```python
from build123d import *

# Parameters (mm, degrees)
BOSS_EXTRUDE1_DEPTH   = 79.375
BOSS_EXTRUDE1_2_DEPTH = 79.375
BOSS_EXTRUDE2_DEPTH   = 3.175
BOSS_EXTRUDE3_START   = 3.175
BOSS_EXTRUDE3_DEPTH   = 3.175


with BuildPart() as part:
    # Sketch2 → Boss-Extrude1 (new body)
    with BuildSketch(Plane.XY):
        with BuildLine():
            Line((0, 304.8), (0, 307.975))
            ThreePointArc((0, 307.975), (-56.126600757, 284.726600757), (-79.375, 228.6))
            Line((-79.375, 228.6), (-79.375, 76.2))
            ThreePointArc((-79.375, 76.2), (-63.5, 28.575), (-22.225, 0))
            Line((-22.225, 0), (0, 0))
            ThreePointArc((0, 0), (-53.881536726, 22.318463274), (-76.2, 76.2))
            Line((-76.2, 76.2), (-76.2, 228.6))
            ThreePointArc((-76.2, 228.6), (-53.881536726, 282.481536726), (0, 304.8))
        make_face()
    extrude(amount=BOSS_EXTRUDE1_DEPTH)



with BuildPart() as body_2:
    # Sketch2 → Boss-Extrude1 2 (new body)
    with BuildSketch(Plane.XY):
        with BuildLine():
            ThreePointArc((-48.2, 88.2), (-34.082546853, 54.117453147), (0, 40))
            Line((0, 40), (0, 43.175))
            ThreePointArc((0, 43.175), (-31.837482823, 56.362517177), (-45.025, 88.2))
            Line((-45.025, 88.2), (-45.025, 216.6))
            ThreePointArc((-45.025, 216.6), (-31.837482823, 248.437482823), (0, 261.625))
            Line((0, 261.625), (0, 264.8))
            ThreePointArc((0, 264.8), (-34.082546853, 250.682546853), (-48.2, 216.6))
            Line((-48.2, 216.6), (-48.2, 88.2))
        make_face()
    extrude(amount=BOSS_EXTRUDE1_2_DEPTH)


with BuildPart() as part_1:
    add(part.part)

    add(body_2.part)  # Boss-Extrude2 merges body 2
    # Sketch3 → Boss-Extrude2 (add)
    with BuildSketch(Plane.XY.offset(79.375)):
        with BuildLine():
            Line((-45.025, 88.2), (-45.025, 216.6))
            ThreePointArc((-45.025, 216.6), (-31.837482823, 248.437482823), (0, 261.625))
            Line((0, 261.625), (0, 307.975))
            ThreePointArc((0, 307.975), (-56.126600757, 284.726600757), (-79.375, 228.6))
            Line((-79.375, 228.6), (-79.375, 76.2))
            ThreePointArc((-79.375, 76.2), (-63.5, 28.575), (-22.225, 0))
            Line((-22.225, 0), (0, 0))
            Line((0, 0), (0, 43.175))
            ThreePointArc((0, 43.175), (-31.837482823, 56.362517177), (-45.025, 88.2))
        make_face()
    extrude(amount=BOSS_EXTRUDE2_DEPTH)

    # Sketch4 → Boss-Extrude3 (add)
    with BuildSketch(Plane(origin=(0, 0, 0), x_dir=(-1, 0, 0), z_dir=(0, 0, -1)).offset(BOSS_EXTRUDE3_START)):
        with BuildLine():
            Line((79.375, 76.2), (79.375, 228.6))
            ThreePointArc((79.375, 228.6), (56.126600757, 284.726600757), (0, 307.975))
            Line((0, 307.975), (0, 261.625))
            ThreePointArc((0, 261.625), (31.837482823, 248.437482823), (45.025, 216.6))
            Line((45.025, 216.6), (45.025, 88.2))
            ThreePointArc((45.025, 88.2), (31.837482823, 56.362517177), (0, 43.175))
            Line((0, 43.175), (0, 0))
            Line((0, 0), (22.225, 0))
            ThreePointArc((22.225, 0), (63.5, 28.575), (79.375, 76.2))
        make_face()
    extrude(amount=-BOSS_EXTRUDE3_DEPTH)


solid = part_1.part
```
Model file for the job. Use its own axes, mm. A direction names the side the tool comes from. Round coordinates to 2 decimals unless told otherwise and drop trailing zeros. Write each loop counter-clockwise with the first axis right and the second up, starting at its lowest first coordinate (ties: lowest second). Pieces come first, ordered by that corner, then holes. Notation, with made-up numbers: (9.5, 87.5) - (62.5, 87.5) arc R22 ccw to (62.5, 123.5) - close; hole circle Ø8 at (42.25, 78). An arc over 180 degrees is marked (long way). Use CSV: the item, a comma, the result in double quotes. Start each with the question number.
Item 1: Band-saw the part on B-B (y = 124). Write the cut outline in (x, z) (3 decimals), and give its area (3 significant figures).
Item 2: Two-plate mould, pull along Y, no slides. Class faces 4 (the face through (-63.068, 28.005, 39.087)), 5 (the face through (-32.186, 56.715, 39.087)), 6 (the face through (-49, 156, 82.55)), 7 (the face through (-56, 155, 79.375)): released by +Y, released by -Y, zero draft, split by the parting line, or undercut.
Item 3: Band-saw the part on C-C (z = 69.5). Write the cut outline in (x, y) (3 decimals), and give its area (3 significant figures).
Item 4: Tool access for faces 1 (the face through (-31.485, 248.786, 39.087)), 2 (the face through (-53.286, 21.729, 39.132)), 3 (the face through (0, 306, 36)): list every direction of +Z, -Z, +X, -X, +Y, -Y with a clear straight run to the whole face (end or side of a thin tool).
Item 5: Band-saw the part on D-D (x = -18.5). Write the cut outline in (y, z) (3 decimals), and give its area (3 significant figures).
Item 6: Pin check, flat tips, straight feed: P1, Ø8, axis at x = -16.5, z = 40.5, coming from the +Y side; P2, Ø24, axis at y = 170, z = 51.5, coming from the +X side (3 decimals); P3, Ø6, axis at x = -42.5, z = 69, coming from the -Y side. Stop position of each tip, or through.
Item 7: Drill centre lines: L1, parallel to Z at x = -63, y = 107.5 (3 decimals); L2, parallel to Y at x = -32.5, z = 74.5; L3, parallel to X at y = 142, z = 61 (3 decimals). Where is each one in solid material? Low to high. Write a range as [from, to].
Item 8: Band-saw the part on A-A (x = -37). Write the cut outline in (y, z) (3 decimals).
Checked values:
1,outline,"(-79.375, -3.175) - (-45.025, -3.175) - (-45.025, 82.55) - (-79.375, 82.55) - close; hole (-76.2, 0) - (-48.2, 0) - (-48.2, 79.375) - (-76.2, 79.375) - close"
1,area,"722 mm²"
2,face 4,"released by -Y"
2,face 5,"undercut"
2,face 6,"zero draft"
2,face 7,"undercut"
3,outline,"(-79.375, 76.2) arc R79.375 ccw to (-22.225, 0) - (0, 0) arc R76.2 cw to (-76.2, 76.2) - (-76.2, 228.6) arc R76.2 cw to (0, 304.8) - (0, 307.975) arc R79.375 ccw to (-79.375, 228.6) - close; (-48.2, 88.2) arc R48.2 ccw to (0, 40) - (0, 43.175) arc R45.025 cw to (-45.025, 88.2) - (-45.025, 216.6) arc R45.025 cw to (0, 261.625) - (0, 264.8) arc R48.2 ccw to (-48.2, 216.6) - close"
3,area,"2,090 mm²"
4,face 1,"+Z, -Z, +X"
4,face 2,"none"
4,face 3,"+Z, -Z, +X, +Y, -Y"
5,outline,"(0, -3.175) - (47.151, -3.175) - (47.151, 82.55) - (0, 82.55) - close; (257.649, -3.175) - (305.789, -3.175) - (305.789, 82.55) - (257.649, 82.55) - close; hole (2.28, 0) - (43.692, 0) - (43.692, 79.375) - (2.28, 79.375) - close; hole (261.108, 0) - (302.52, 0) - (302.52, 79.375) - (261.108, 79.375) - close"
5,area,"1,590 mm²"
6,P1,"stops at y = 306.98"
6,P2,"stops at x = -45.025"
6,P3,"stops at y = 7.35"
7,L1,"z = [-3.175, 0], [79.375, 82.55]"
7,L2,"y = [3.78, 7.28], [52.61, 57.04], [247.76, 252.19], [297.52, 301.02]"
7,L3,"x = [-79.375, -76.2], [-48.2, -45.025]"
8,outline,"(5.976, -3.175) - (62.544, -3.175) - (62.544, 82.55) - (5.976, 82.55) - close; (242.256, -3.175) - (298.824, -3.175) - (298.824, 82.55) - (242.256, 82.55) - close; hole (9.586, 0) - (57.309, 0) - (57.309, 79.375) - (9.586, 79.375) - close; hole (247.491, 0) - (295.214, 0) - (295.214, 79.375) - (247.491, 79.375) - close"
